Verification items for the finished model (mm, model axes). A direction names the side the tool comes from. Round coordinates to 2 decimals unless told otherwise and drop trailing zeros. Order: outer loops, then holes, each group sorted by start corner. A loop starts at its lowest first (then second) coordinate and runs counter-clockwise, first axis right, second up. Notation, with made-up numbers: (16, 62.5) -> (43, 62.5) arc R28 cw to (43, 99.5) -> close; hole circle Ø7 at (-31.5, 74). An arc over 180 degrees is marked (long way). Put each result on its own line as item: value.
from build123d import *

# Parameters (mm, degrees)
F0_W     = 1200
F0_H     = 600
F1_DEPTH = 70
F2_T     = -2.5
F3_R     = 5
F4_R     = 5


with BuildPart() as f1:
    # F0 (on Top) → F1 (new body)
    with BuildSketch(Plane.XY):
        with Locations((600, 300)):
            Rectangle(F0_W, F0_H)
    extrude(amount=F1_DEPTH)

    # F2
    f2_openings = [f1.faces().sort_by_distance(p)[0] for p in [
        (600, 300, 70),
    ]]
    offset(amount=F2_T, openings=f2_openings)

    # F3
    f3_edges = [f1.edges().sort_by_distance(p)[0] for p in [
        (0, 300, 0),
        (600, 0, 0),
        (1200, 300, 0),
        (600, 600, 0),
    ]]
    fillet(f3_edges, radius=F3_R)

    # F4
    f4_edges = [f1.edges().sort_by_distance(p)[0] for p in [
        (2.5, 300, 2.5),
        (600, 2.5, 2.5),
        (1197.5, 300, 2.5),
        (600, 597.5, 2.5),
    ]]
    fillet(f4_edges, radius=F4_R)


solid = f1.part
Item 1: Tool access check on faces 4 (the flat face through (592, 2.5, 38)), 5 (the flat face through (1200, 296, 37)). Record the directions out of +Z, -Z, +X, -X, +Y, -Y that give a thin tool (end or side, any length) a straight path to the whole face; none if there is none.
Check sheet entries:
face 4: +Z
face 5: +Z, -Z, +X, +Y, -Y
Item 2: Section check C-C on x = 597. Record the boundary of the cut face in (y, z), then the cut area to 3 significant figures.
Check sheet entries:
outline: (0, 5) arc R5 ccw to (5, 0) -> (595, 0) arc R5 ccw to (600, 5) -> (600, 70) -> (597.5, 70) -> (597.5, 7.5) arc R5 cw to (592.5, 2.5) -> (7.5, 2.5) arc R5 cw to (2.5, 7.5) -> (2.5, 70) -> (0, 70) -> close
area: 1,840 mm^2
Item 3: Release check for a two-part mould opening along Y. For faces 1 (the flat face through (592, 600, 37)), 2 (the flat face through (0, 296, 37)), 3 (the flat face through (592, 304, 2.5)) record: +Y half, -Y half, draft (parallel to the pull), parting line (faces both ways), or undercut.
Check sheet entries:
face 1: +Y half
face 2: draft
face 3: undercut
Item 4: Material ranges on L1, parallel to Y at x = 172.5, z = 22; L2, parallel to X at y = 281, z = 42; L3, parallel to X at y = 106.5, z = 6, recorded low to high. Write a range as [from, to].
Check sheet entries:
L1: y = [0, 2.5], [597.5, 600]
L2: x = [0, 2.5], [1197.5, 1200]
L3: x = [0, 2.73], [1197.27, 1200]
Item 5: Section check A-A on z = 30. Record the boundary of the cut face in (x, y), then the cut area to 4 significant figures.
Check sheet entries:
outline: (0, 0) -> (1200, 0) -> (1200, 600) -> (0, 600) -> close; hole (2.5, 2.5) -> (1197.5, 2.5) -> (1197.5, 597.5) -> (2.5, 597.5) -> close
area: 8,975 mm^2
Item 6: Gauge pin test, flat ends, axial feed: pin 1 Ø12 at (x, y) = (818.5, 403) entering from +Z; pin 2 Ø1 at (x, z) = (294, 60) entering from -Y. Record the tip position at first contact, or that the pin passes through.
Check sheet entries:
pin 1: stops at z = 2.5
pin 2: stops at y = 0
Item 7: Section check B-B on y = 388.5. Record the boundary of the cut face in (x, z), then the cut area to 3 significant figures.
Check sheet entries:
outline: (0, 5) arc R5 ccw to (5, 0) -> (1195, 0) arc R5 ccw to (1200, 5) -> (1200, 70) -> (1197.5, 70) -> (1197.5, 7.5) arc R5 cw to (1192.5, 2.5) -> (7.5, 2.5) arc R5 cw to (2.5, 7.5) -> (2.5, 70) -> (0, 70) -> close
area: 3,340 mm^2
